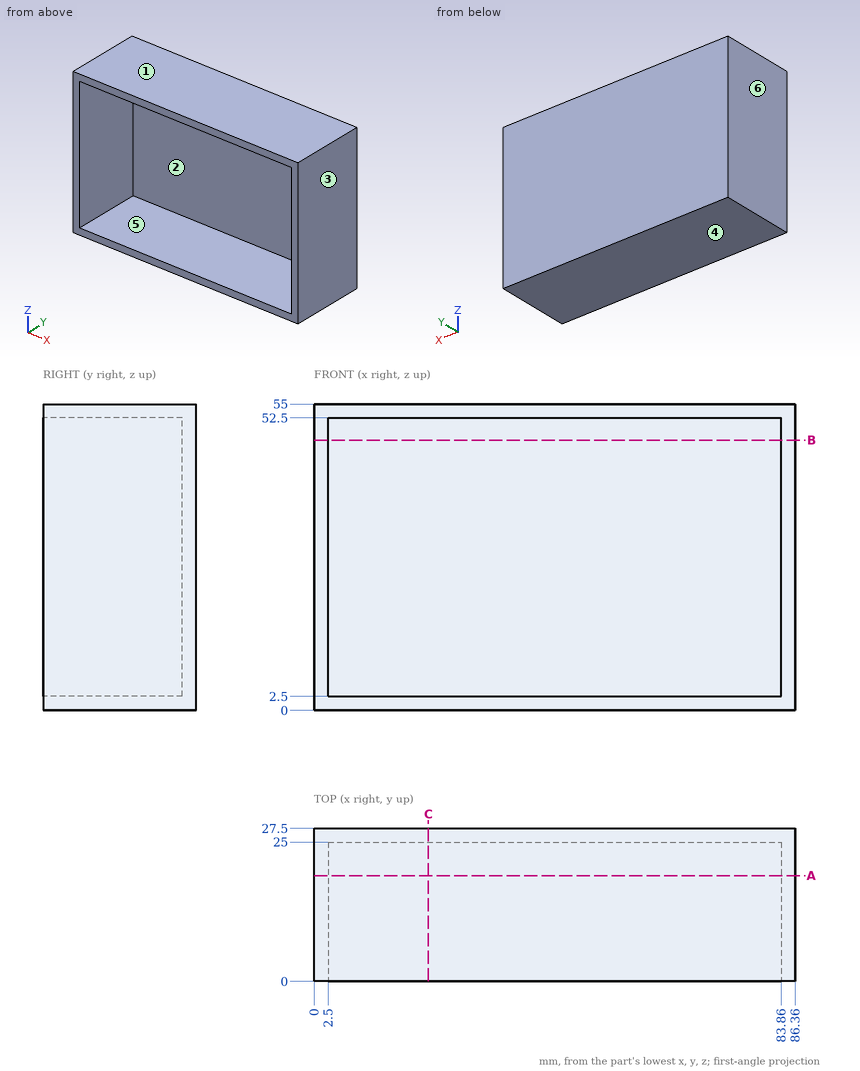
Design review of the part shown in the three views and the two pictorial views. Dimensions are in mm from the part's minimum x, y and z. A direction names the side the tool comes from. Round coordinates to 2 decimals unless told otherwise and drop trailing zeros. Loops run counter-clockwise (first coordinate to the right, second up) from the corner with the lowest first, then second, coordinate; pieces in that order, holes last. Notation, with made-up numbers: (16.25, 52) -> (20.25, 52) arc R17 ccw to (20.25, 85) -> close; hole circle Ø8 at (52, 86.5). An arc over 180 degrees is marked (long way). Answer as a JSON object with one key per item and string values. Group by question number.
1) We need section A-A on y = 19. Write out the cut boundary in (x, z).
2) For line 1 (X direction, y = 22, z = 31.5); line 2 (Z direction, x = 73.5, y = 24.25); line 3 (Y direction, x = 52, z = 51), list the stretches that pass through material, from the lowest coordinate up. Write a range as [from, to].
3) We need section C-C on x = 20.5. Write out the cut boundary in (y, z).
4) Mouldability with a two-part tool opening along Z and no side actions: class the marked faces 1, 2, 3 and 4 as released by +Z, released by -Z, zero draft, split by the parting line, or undercut.
5) For pin 1 Ø4 at (x, z) = (34, 17.5) entering from -Y, flat-tipped, find the tip position at first contact; note if it passes through.
6) For the marked faces 5 and 6, list the 3-axis set-ups (+Z, -Z, +X, -X, +Y, -Y) from which the entire face can be reached by the end or side of a thin tool; tool diameter is ignored.
7) We need section B-B on z = 48.5. Write out the cut boundary in (x, y), then the cut area to 3 significant figures.
Result set:
{
 "1": {"outline": "(0, 0) -> (86.36, 0) -> (86.36, 55) -> (0, 55) -> close; hole (2.5, 2.5) -> (83.86, 2.5) -> (83.86, 52.5) -> (2.5, 52.5) -> close"},
 "2": {"line 1": "[0, 2.5], [83.86, 86.36]", "line 2": "[0, 2.5], [52.5, 55]", "line 3": "[25, 27.5]"},
 "3": {"outline": "(0, 0) -> (27.5, 0) -> (27.5, 55) -> (0, 55) -> (0, 52.5) -> (25, 52.5) -> (25, 2.5) -> (0, 2.5) -> close"},
 "4": {"face 1": "released by +Z", "face 2": "undercut", "face 3": "zero draft", "face 4": "released by -Z"},
 "5": {"pin 1": "y = 25"},
 "6": {"face 5": "-Y", "face 6": "+Z, -Z, -X, +Y, -Y"},
 "7": {"outline": "(0, 0) -> (2.5, 0) -> (2.5, 25) -> (83.86, 25) -> (83.86, 0) -> (86.36, 0) -> (86.36, 27.5) -> (0, 27.5) -> close", "area": "341 mm²"}
}
